Print and shaded views of the part. All mm, measured from the part's lowest x, y and z. A direction names the side the tool comes from. Coordinates: 2 decimals unless noted, no trailing zeros. Order: outer loops, then holes, each group sorted by start corner. A loop starts at its lowest first (then second) coordinate and runs counter-clockwise, first axis right, second up. Notation, with made-up numbers: (-12, 27.25) - (0, 27.25) arc R30 cw to (0, 62.25) - close; hole circle Ø2 at (83, 11.5). An arc over 180 degrees is marked (long way). Write each question's results on one line, items separated by ' | '.
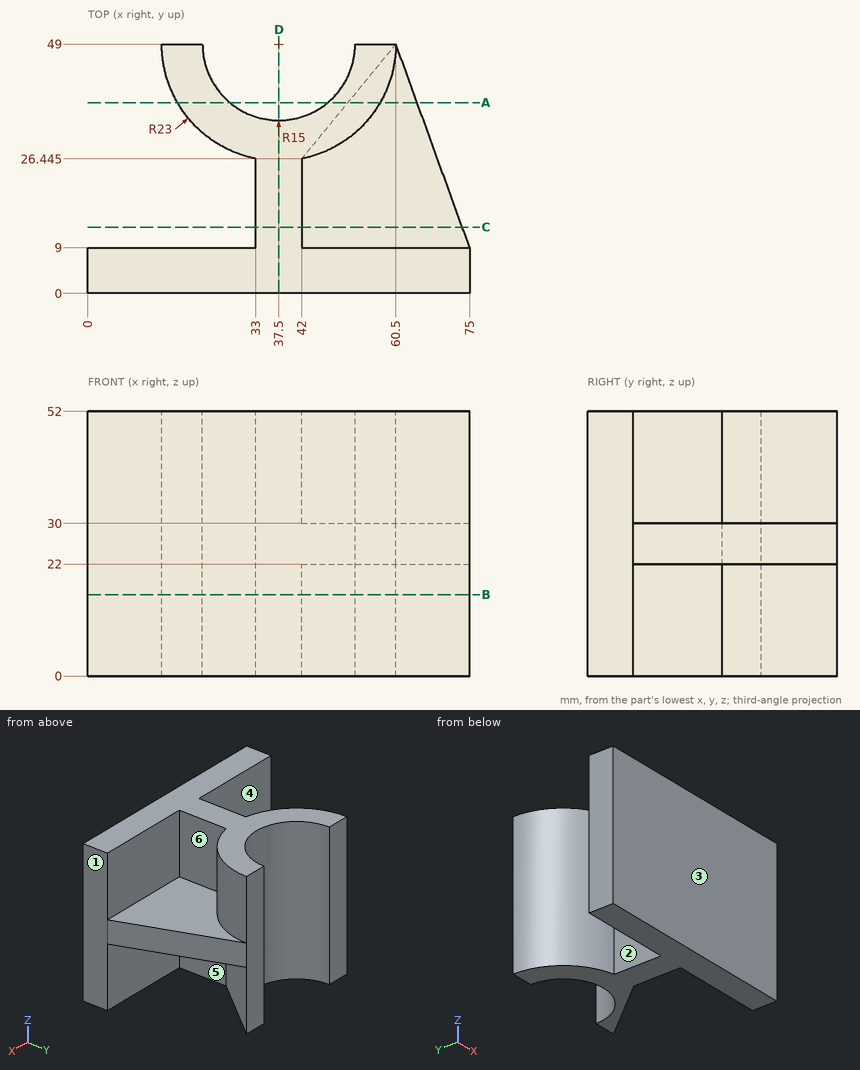
1. Band-saw the part on D-D on x = 37.5. Give the cut face in (y, z), then the cut area to 3 significant figures.
Solved:
outline: (0, 0) - (34, 0) - (34, 52) - (0, 52) - close | area: 1,770 mm2
2. Probe line 1 (Z direction, x = 44, y = 24); line 2 (X direction, y = 46, z = 46); line 3 (Y direction, x = 8.5, z = 13). List the from-to ranges inside material, lowest first.
Solved:
line 1: z = 22 to 30 | line 2: x = 14.7 to 22.8, 52.2 to 60.3 | line 3: y = 0 to 9
3. Band-saw the part on C-C on y = 13. Give the cut face in (x, z).
Solved:
outline: (33, 0) - (42, 0) - (42, 22) - (73.55, 22) - (73.55, 30) - (42, 30) - (42, 52) - (33, 52) - close
4. Band-saw the part on B-B on z = 16. Give the cut face in (x, y) (1 decimal).
Solved:
outline: (0, 0) - (75, 0) - (75, 9) - (42, 9) - (42, 26.4) - (60.5, 49) - (52.5, 49) arc R15 cw to (22.5, 49) - (14.5, 49) arc R23 ccw to (33, 26.4) - (33, 9) - (0, 9) - close
5. Drop flat-ended pins along their axis: pin 1 Ø1.5 at (y, z) = (44, 9.5) entering from +X (1 decimal); pin 2 Ø5 at (x, y) = (66, 24.5) entering from +Z; pin 3 Ø8.5 at (y, z) = (22, 36) entering from -X. Give the stop position or say it passes through.
Solved:
pin 1: stops at x = 57 | pin 2: stops at z = 30 | pin 3: stops at x = 33
6. Two-plate mould, pull along Y, no slides. Class the marked faces 1, 2 and 3: +Y half, -Y half, draft (parallel to the pull), parting line (faces both ways), or undercut.
Solved:
face 1: draft | face 2: undercut | face 3: -Y half
7. Tool access for the marked faces 4, 5 and 6: list every direction of +Z, -Z, +X, -X, +Y, -Y with a clear straight run to the whole face (end or side of a thin tool).
Solved:
face 4: +Z, -Z, -X | face 5: -Z, +X | face 6: +Z, +X
8. Band-saw the part on A-A on y = 37.5. Give the cut face in (x, z), then the cut area to 3 significant figures.
Solved:
outline: (17.58, 0) - (27.87, 0) - (27.87, 52) - (17.58, 52) - close; (47.13, 0) - (51.07, 0) - (51.07, 22) - (64.67, 22) - (64.67, 30) - (57.42, 30) - (57.42, 52) - (47.13, 52) - close | area: 988 mm2
